Verification items for this drawing (mm, ordinates from the low corner). Round coordinates to 2 decimals unless told otherwise and drop trailing zeros. Order: outer loops, then holes, each group sorted by start corner. A loop starts at its lowest first (then second) coordinate and runs counter-clockwise, first axis right, second up. Notation, with made-up numbers: (72, 11) - (80, 11) arc R10 cw to (80, 30) - close; hole circle Ø10 at (80, 71.5). An arc over 180 degrees is marked (long way). Use a Markdown table: item, result. Add a question column.
(1) Mould release check, pull along Z, two halves, no side actions. Record for the marked faces 1 and 2: released by +Z, released by -Z, zero draft, split by the parting line, or undercut.
(2) Section check C-C on z = 4.5. Record the boundary of the cut face in (x, y).
(3) Section check B-B on x = 2. Record the boundary of the cut face in (y, z) (1 decimal).
(4) Section check A-A on x = 5.5. Record the boundary of the cut face in (y, z) (1 decimal).
(5) Thickness scan on line 1 along Z through (x, y) = (7.75, 0.45); line 2 along X through (y, z) = (0.15, 10.5). Record the ranges inside material, lowest first. Write a range as [from, to].
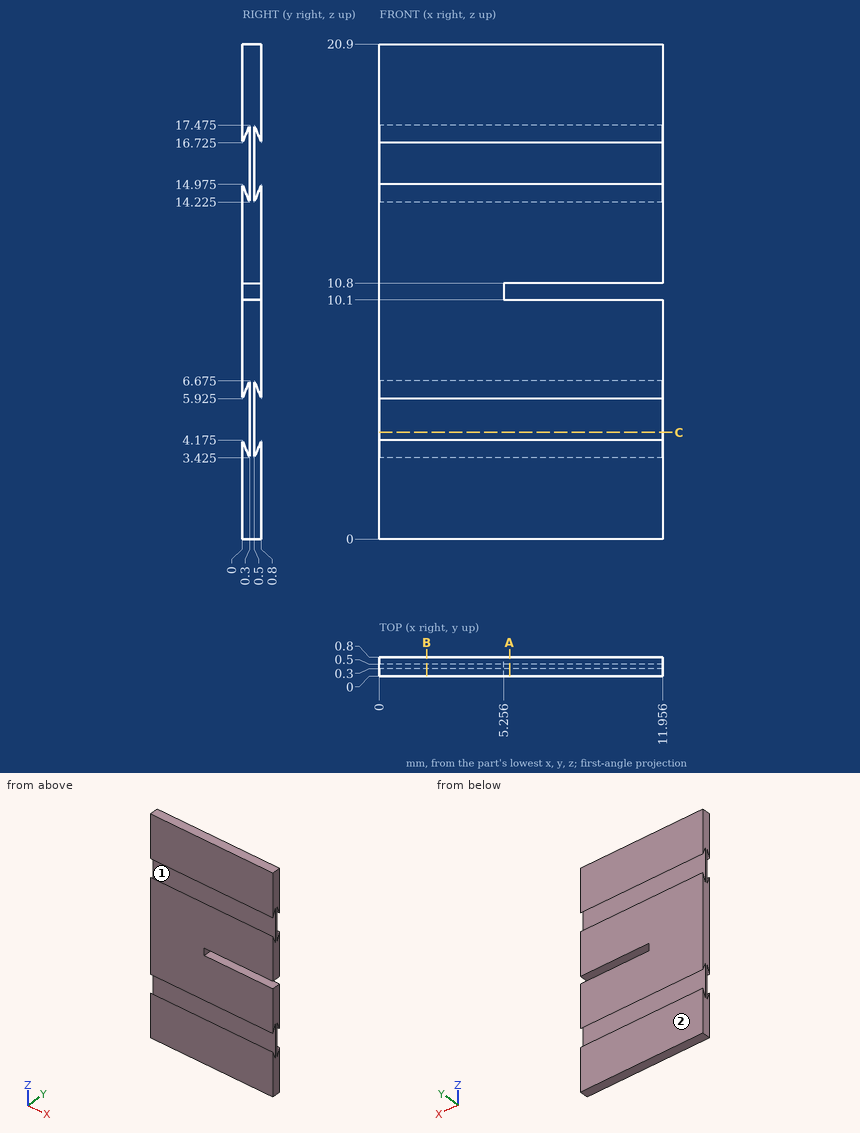
Check sheet entries:
| question | item | result |
|---|---|---|
| 1 | face 1 | undercut |
| 1 | face 2 | zero draft |
| 2 | outline | (0, 0.3) - (11.96, 0.3) - (11.96, 0.5) - (0, 0.5) - close |
| 3 | outline | (0, 0) - (0.8, 0) - (0.8, 4.2) - (0.5, 3.4) - (0.5, 6.7) - (0.8, 5.9) - (0.8, 15) - (0.5, 14.2) - (0.5, 17.5) - (0.8, 16.7) - (0.8, 20.9) - (0, 20.9) - (0, 16.7) - (0.3, 17.5) - (0.3, 14.2) - (0, 15) - (0, 5.9) - (0.3, 6.7) - (0.3, 3.4) - (0, 4.2) - close |
| 4 | outline | (0, 0) - (0.8, 0) - (0.8, 4.2) - (0.5, 3.4) - (0.5, 6.7) - (0.8, 5.9) - (0.8, 10.1) - (0, 10.1) - (0, 5.9) - (0.3, 6.7) - (0.3, 3.4) - (0, 4.2) - close; (0, 10.8) - (0.8, 10.8) - (0.8, 15) - (0.5, 14.2) - (0.5, 17.5) - (0.8, 16.7) - (0.8, 20.9) - (0, 20.9) - (0, 16.7) - (0.3, 17.5) - (0.3, 14.2) - (0, 15) - close |
| 5 | line 1 | z = [0, 10.1], [10.8, 20.9] |
| 5 | line 2 | x = [0, 5.26] |
